Autodesk Inventor part; units mm, degrees
ref_plane "YZ Plane" through (0, 0, 0) normal (1, 0, 0) x (0, 1, 0)
ref_plane "XZ Plane" through (0, 0, 0) normal (0, 1, 0) x (-1, 0, 0)
ref_plane "XY Plane" through (0, 0, 0) normal (0, 0, 1) x (1, 0, 0)
sketch "Sketch1" plane through (0, 0, 0) normal (0, 1, 0) x (-1, 0, 0)
  line L0 (0, 0) -> (-44.45, 0)
  line L1 (-44.45, 0) -> (-44.45, -47.5996)
  line L2 (-44.45, -47.5996) -> (0, -47.5996)
  line L3 (0, -47.5996) -> (0, 0)
  dimension "d0" = 44.45
  dimension "d1" = 47.5996
extrude "Extrusion1" add sketch "Sketch1" along normal blind 6.35
sketch "Sketch2" plane through (0, 6.35, 0) normal (0, 1, 0) x (1, 0, 0)
  line L0 (0, 47.5996) -> (0, 0)
  line L1 (0, 12.7) -> (6.35, 12.7)
  line L2 (6.35, 12.7) -> (6.35, 34.036)
  line L3 (6.35, 34.036) -> (0, 34.036)
  line L4 (0, 34.036) -> (0, 12.7)
  line L5 (44.45, 0) -> (44.45, 47.5996)
  line L6 (44.45, 12.7) -> (38.1, 12.7)
  line L7 (38.1, 12.7) -> (38.1, 34.036)
  line L8 (38.1, 34.036) -> (44.45, 34.036)
  line L9 (44.45, 34.036) -> (44.45, 12.7)
  dimension "d4" = 6.35
  dimension "d5" = 21.336
  dimension "d6" = 6.35
extrude "Extrusion2" cut sketch "Sketch2" against normal blind 6.35
sketch "Sketch3" plane through (0, 6.35, 0) normal (0, 1, 0) x (1, 0, 0)
  circle A0 centre (22.225, 23.7998) radius 3.175
  circle A1 centre (32.3088, 23.7998) radius 1.27
  circle A2 centre (17.1831, 32.5326) radius 1.27
  circle A3 centre (17.1831, 15.067) radius 1.27
  point P0 (0, 0)
  dimension "d9" = 6.35
  dimension "d10" = 2.54
  dimension "d13" = 360
extrude "Extrusion3" cut sketch "Sketch3" against normal blind 6.35
sketch "Sketch4" plane through (0, 6.35, 0) normal (0, 1, 0) x (1, 0, 0)
  line L0 (44.45, 47.5996) -> (48.26, 47.5996)
  line L1 (48.26, 47.5996) -> (48.26, 0)
  line L2 (48.26, 0) -> (44.45, 0)
  line L3 (44.45, 0) -> (44.45, 47.5996)
  line L4 (0, 47.5996) -> (-3.81, 47.5996)
  line L5 (-3.81, 47.5996) -> (-3.81, 0)
  line L6 (-3.81, 0) -> (0, 0)
  line L7 (0, 0) -> (0, 47.5996)
  line L8 (0, 12.7) -> (6.35, 12.7)
  line L9 (6.35, 34.036) -> (2.54, 34.036)
  line L10 (2.54, 34.036) -> (2.54, 12.7)
  line L11 (2.54, 12.7) -> (6.35, 12.7)
  line L12 (6.35, 12.7) -> (6.35, 34.036)
  line L13 (44.45, 12.7) -> (38.1, 12.7)
  line L14 (38.1, 34.036) -> (41.91, 34.036)
  line L15 (41.91, 34.036) -> (41.91, 12.7)
  line L16 (41.91, 12.7) -> (38.1, 12.7)
  line L17 (38.1, 12.7) -> (38.1, 34.036)
  point P0 (0, 0)
  dimension "d17" = 3.81
  dimension "d18" = 3.81
  dimension "d19" = 3.81
  dimension "d20" = 3.81
extrude "Extrusion4" add sketch "Sketch4" against normal blind 6.35
sketch "Sketch5" plane through (0, 6.35, 0) normal (0, 1, 0) x (1, 0, 0)
  line L0 (-3.81, 0) -> (-3.81, 47.5996)
  line L1 (0, 34.036) -> (-3.81, 34.036)
  line L2 (-3.81, 34.036) -> (-3.81, 12.7)
  line L3 (-3.81, 12.7) -> (0, 12.7)
  line L4 (0, 12.7) -> (0, 34.036)
  line L5 (48.26, 47.5996) -> (48.26, 0)
  line L6 (44.45, 34.036) -> (48.26, 34.036)
  line L7 (48.26, 34.036) -> (48.26, 12.7)
  line L8 (48.26, 12.7) -> (44.45, 12.7)
  line L9 (44.45, 12.7) -> (44.45, 34.036)
  point P0 (0, 0)
extrude "Extrusion5" cut sketch "Sketch5" against normal blind 6.35
sketch "Sketch6" plane through (0, 6.35, 0) normal (0, 1, 0) x (1, 0, 0)
  line L0 (48.26, 12.7) -> (48.26, 0)
  line L1 (-3.81, 0) -> (48.26, 0)
  line L2 (48.26, 0) -> (48.26, 1.27)
  line L3 (48.26, 1.27) -> (-3.81, 1.27)
  line L4 (-3.81, 1.27) -> (-3.81, 0)
  line L5 (48.26, 47.5996) -> (48.26, 34.036)
  line L6 (-3.81, 47.5996) -> (48.26, 47.5996)
  line L7 (48.26, 47.5996) -> (48.26, 46.736)
  line L8 (48.26, 46.736) -> (-3.81, 46.736)
  line L9 (-3.81, 46.736) -> (-3.81, 47.5996)
  point P0 (0, 0)
  dimension "d25" = 1.27
  dimension "d26" = 0.8636
extrude "Extrusion6" cut sketch "Sketch6" against normal blind 25.4
properties part number "motor holder"
Here's how the part is built. I have some questions about the finished solid (model axes, mm). A direction names the side the tool comes from. Give positions to 0.01 mm unless a question says otherwise; leave off trailing zeros. Write each loop counter-clockwise with the first axis right and the second up, starting at its lowest first coordinate (ties: lowest second). Pieces come first, ordered by that corner, then holes. Notation, with made-up numbers: M 18,75.25 L 68,75.25 A20 cw 68,89.25 Z; hole C 29,15.5 d8. An arc over 180 degrees is marked long. Put each result on its own line as item: value. Start each with the question number.
Item 1: On a 3-axis mill with a long thin cutter (end or side, diameter ignored), from which of +Z, -Z, +X, -X, +Y, -Y can I reach the whole of each face in a straight line? I mean faces 4 (the flat face through (45, 3, -12.7)), 5 (the flat face through (-1, 3, -12.7)), 6 (the flat face through (-3.81, 3, -40)). Say none if no direction works.
Item 2: If we section it at A-A, the plane x = 43: Write out the boundary of the cut face in (y, z), then the cut area to 3 significant figures.
Item 3: Thinking about a two-plate mould opening in X: for faces 1 (the cylindrical face through (16.175, 3.219, -31.76)), 2 (the flat face through (45, 3, -34.036)), 3 (the flat face through (2.54, 3, -24)), which applies, +X half, -X half, draft (parallel to the pull), parting line (faces both ways), or undercut?
Item 4: Will these pins go through, and if not, where does the flat tip stop? pin 1 (1.9 mm diameter, centred on y = 4.5, z = -21, fed in from +X); pin 2 (1.9 mm diameter, centred on y = 4, z = -23.5, fed in from -X).
Item 5: If we section it at C-C, the plane z = -26: Write out the boundary of the cut face in (x, y), then the cut area to 3 significant figures.
Item 6: I need wall thicknesses on L1, parallel to X at y = 2, z = -24; L2, parallel to X at y = 1.5, z = -23.5; L3, parallel to Z at x = 23, y = 5.5. Which ranges of each line are inside material? Lowest first, please. Write a range as from..to.
Item 7: If we section it at B-B, the plane y = 2.25: Write out the boundary of the cut face in (x, z) (3 decimals), then the cut area to 3 significant figures.
Values:
1. face 4: +X, +Y, -Y
1. face 5: -X, +Y, -Y
1. face 6: +Z, -Z, -X, +Y, -Y
2. outline: M 0,-46.74 L 6.35,-46.74 L 6.35,-34.04 L 0,-34.04 Z; M 0,-12.7 L 6.35,-12.7 L 6.35,-1.27 L 0,-1.27 Z
2. area: 153 mm²
3. face 1: undercut
3. face 2: draft
3. face 3: -X half
4. pin 1: x = 41.91
4. pin 2: x = 2.54
5. outline: M 2.54,0 L 19.94,0 L 19.94,6.35 L 2.54,6.35 Z; M 24.51,0 L 41.91,0 L 41.91,6.35 L 24.51,6.35 Z
5. area: 221 mm²
6. L1: 2.54..19.06, 25.39..31.05, 33.56..41.91
6. L2: 2.54..19.06, 25.39..31.07, 33.54..41.91
6. L3: -46.74..-26.88, -20.72..-1.27
7. outline: M -3.81,-46.736 L 48.26,-46.736 L 48.26,-34.036 L 41.91,-34.036 L 41.91,-12.7 L 48.26,-12.7 L 48.26,-1.27 L -3.81,-1.27 L -3.81,-12.7 L 2.54,-12.7 L 2.54,-34.036 L -3.81,-34.036 Z; hole C 17.183,-32.533 d2.54; hole C 17.183,-15.067 d2.54; hole C 22.225,-23.8 d6.35; hole C 32.309,-23.8 d2.54
7. area: 2,050 mm²
